```python
from build123d import *

# Parameters (mm, degrees)
CUT_EXTRUDE2_REACH = 107.371
SKETCH3_R          = 3.175


with BuildPart() as part:
    # Sketch1 → Revolve1 (revolve)
    with BuildSketch(Plane.XY):
        Polygon((0, 7.9375), (72.324156056, 50.8), (-20.347266862, 50.8), (-20.347266862, 69.85), (-33.047266862, 69.85), (-33.047266862, 50.8), (-33.047266862, 41.275), (-12.7, 7.9375), align=None)
    revolve(axis=Axis((0, 0, 0), (1, 0, 0)))

    # Sketch3 → Cut-Extrude2 (cut, up to next)
    with BuildSketch(Plane.ZY.offset(33.047266862), mode=Mode.PRIVATE) as cut_extrude2_sk1:
        with Locations((0, 59.9186)):
            Circle(SKETCH3_R)
    cut_extrude2_tool1 = extrude(cut_extrude2_sk1.sketch, amount=-CUT_EXTRUDE2_REACH, mode=Mode.PRIVATE) & part.part
    add(cut_extrude2_tool1.solids().sort_by_distance((-33.047267, 59.9186, 0))[0], mode=Mode.SUBTRACT)
    # Sketch3 → Cut-Extrude2 (cut, up to next)
    with BuildSketch(Plane.ZY.offset(33.047266862), mode=Mode.PRIVATE) as cut_extrude2_sk2:
        with Locations((42.368848379, 42.368848379)):
            Circle(SKETCH3_R)
    cut_extrude2_tool2 = extrude(cut_extrude2_sk2.sketch, amount=-CUT_EXTRUDE2_REACH, mode=Mode.PRIVATE) & part.part
    add(cut_extrude2_tool2.solids().sort_by_distance((-33.047267, 42.368848, 42.368848))[0], mode=Mode.SUBTRACT)
    # Sketch3 → Cut-Extrude2 (cut, up to next)
    with BuildSketch(Plane.ZY.offset(33.047266862), mode=Mode.PRIVATE) as cut_extrude2_sk3:
        with Locations((59.9186, 0)):
            Circle(SKETCH3_R)
    cut_extrude2_tool3 = extrude(cut_extrude2_sk3.sketch, amount=-CUT_EXTRUDE2_REACH, mode=Mode.PRIVATE) & part.part
    add(cut_extrude2_tool3.solids().sort_by_distance((-33.047267, 0, 59.9186))[0], mode=Mode.SUBTRACT)
    # Sketch3 → Cut-Extrude2 (cut, up to next)
    with BuildSketch(Plane.ZY.offset(33.047266862), mode=Mode.PRIVATE) as cut_extrude2_sk4:
        with Locations((42.368848379, -42.368848379)):
            Circle(SKETCH3_R)
    cut_extrude2_tool4 = extrude(cut_extrude2_sk4.sketch, amount=-CUT_EXTRUDE2_REACH, mode=Mode.PRIVATE) & part.part
    add(cut_extrude2_tool4.solids().sort_by_distance((-33.047267, -42.368848, 42.368848))[0], mode=Mode.SUBTRACT)
    # Sketch3 → Cut-Extrude2 (cut, up to next)
    with BuildSketch(Plane.ZY.offset(33.047266862), mode=Mode.PRIVATE) as cut_extrude2_sk5:
        with Locations((0, -59.9186)):
            Circle(SKETCH3_R)
    cut_extrude2_tool5 = extrude(cut_extrude2_sk5.sketch, amount=-CUT_EXTRUDE2_REACH, mode=Mode.PRIVATE) & part.part
    add(cut_extrude2_tool5.solids().sort_by_distance((-33.047267, -59.9186, 0))[0], mode=Mode.SUBTRACT)
    # Sketch3 → Cut-Extrude2 (cut, up to next)
    with BuildSketch(Plane.ZY.offset(33.047266862), mode=Mode.PRIVATE) as cut_extrude2_sk6:
        with Locations((-42.368848379, -42.368848379)):
            Circle(SKETCH3_R)
    cut_extrude2_tool6 = extrude(cut_extrude2_sk6.sketch, amount=-CUT_EXTRUDE2_REACH, mode=Mode.PRIVATE) & part.part
    add(cut_extrude2_tool6.solids().sort_by_distance((-33.047267, -42.368848, -42.368848))[0], mode=Mode.SUBTRACT)
    # Sketch3 → Cut-Extrude2 (cut, up to next)
    with BuildSketch(Plane.ZY.offset(33.047266862), mode=Mode.PRIVATE) as cut_extrude2_sk7:
        with Locations((-59.9186, 0)):
            Circle(SKETCH3_R)
    cut_extrude2_tool7 = extrude(cut_extrude2_sk7.sketch, amount=-CUT_EXTRUDE2_REACH, mode=Mode.PRIVATE) & part.part
    add(cut_extrude2_tool7.solids().sort_by_distance((-33.047267, 0, -59.9186))[0], mode=Mode.SUBTRACT)
    # Sketch3 → Cut-Extrude2 (cut, up to next)
    with BuildSketch(Plane.ZY.offset(33.047266862), mode=Mode.PRIVATE) as cut_extrude2_sk8:
        with Locations((-42.368848379, 42.368848379)):
            Circle(SKETCH3_R)
    cut_extrude2_tool8 = extrude(cut_extrude2_sk8.sketch, amount=-CUT_EXTRUDE2_REACH, mode=Mode.PRIVATE) & part.part
    add(cut_extrude2_tool8.solids().sort_by_distance((-33.047267, 42.368848, -42.368848))[0], mode=Mode.SUBTRACT)


solid = part.part
```
Read the model definition and answer for the solid it produces. Units are mm, in the model's axes. A direction names the side the tool comes from. Round coordinates to 2 decimals unless told otherwise and drop trailing zeros. Write each loop counter-clockwise with the first axis right and the second up, starting at its lowest first coordinate (ties: lowest second). Pieces come first, ordered by that corner, then holes. Notation, with made-up numbers: (88, 45) -> (133, 45) arc R31 ccw to (133, 73) -> close; hole circle Ø2 at (-6.75, 84). An arc over 180 degrees is marked (long way). Answer in a Markdown table with one row per item. Add a question column.
1) Find section D-D, the plane x = 37.5. Determine the outline of the cut face in (y, z).
2) Determine the mould class of faces 3 (the face through (25.34, -11.012, -49.592)), 4 (the face through (-26.786, -45.186, 43.834)), 5 (the face through (-33.047, 30, -30)), 6 (the face through (-26.79, 56.82, -0.69)) for opening direction Y: pulls with the +Y half, pulls with the -Y half, needs draft (parallel to the pull), parting line crosses it, or undercut.
3) Find section C-C, the plane x = -6. Determine the outline of the cut face in (y, z) (1 decimal).
4) Consider line 1 (Y direction, x = 53, z = 31.5); line 2 (Z direction, x = 66, y = 7); line 3 (X direction, y = -38, z = 47). Determine where each line is inside the solid, lowest interval first.
5) Which of the six approach directions +Z, -Z, +X, -X, +Y, -Y give full straight-line access (tool end or side, diameter ignored) to faces 1 (the face through (-20.347, -31, -41)), 2 (the face through (-26.79, 0.95, -56.89))?
6) Given P1, Ø2, axis at x = -13, z = 46.5, coming from the -Y side; P2, Ø12, axis at x = 51.5, y = -32, coming from the -Z side; P3, Ø10, axis at y = 0, z = -59.92, coming from the +X side, each flat-ended and moving along its own axis, determine where each tip first touches the part or whether it passes through.
7) Find section A-A, the plane z = 0. State how many separate pieces and enclosed holes the cut face has, and give its area (3 significant figures).
Findings below:
| question | item | result |
|---|---|---|
| 1 | outline | circle Ø101.6 at (0, 0); hole circle Ø60.32 at (0, 0) |
| 2 | face 3 | parting line crosses it |
| 2 | face 4 | undercut |
| 2 | face 5 | needs draft |
| 2 | face 6 | undercut |
| 3 | outline | circle Ø101.6 at (0, 0); hole circle Ø15.9 at (0, 0) |
| 4 | line 1 | -39.85 to -23.58, 23.58 to 39.85 |
| 4 | line 2 | -50.32 to -46.53, 46.53 to 50.32 |
| 4 | line 3 | -33.05 to -20.35 |
| 5 | face 1 | +X |
| 5 | face 2 | +X, -X |
| 6 | P1 | y = -22.59 |
| 6 | P2 | z = -43.64 |
| 6 | P3 | x = -20.35 |
| 7 | separate pieces | 4 |
| 7 | enclosed holes | 0 |
| 7 | area | 5,580 mm² |
